Here's how the part is built. I have some questions about the finished solid (model axes, mm). Face numbers are marked on the shaded views. Give positions to 0.01 mm unless a question says otherwise; leave off trailing zeros. Write each loop counter-clockwise with the first axis right and the second up, starting at its lowest first coordinate (ties: lowest second). Pieces come first, ordered by that corner, then holes. Notation, with made-up numbers: (43.5, -4) - (68.5, -4) arc R30 cw to (68.5, 33) - close; hole circle Ø5 at (50.25, 49). An arc over 180 degrees is marked (long way). One line per item, written item: value. Start each with the question number.
1) Imagine slicing it at A-A on y = -10.5. Write out the boundary of the cut face in (x, z), plus the area to 3 significant figures.
2) Imagine slicing it at B-B on x = 27.5. Write out the boundary of the cut face in (y, z), plus the area to 3 significant figures.
3) Please list where these lines run through material, in increasing order: L1, parallel to Y at x = -64.5, z = 0.5; L2, parallel to Y at x = 27.5, z = 1; L3, parallel to Y at x = -64.5, z = 1.5. Write a range as [from, to].
4) Imagine slicing it at C-C on z = -1.2. Write out the boundary of the cut face in (x, y), plus the area to 3 significant figures.
5) We'd pull the mould along X, two halves only. Please class the marked faces 1 and 2: +X half, -X half, draft (parallel to the pull), parting line (faces both ways), or undercut.
6) I'm going to push a flat-ended pin straight in: P1, Ø8, axis at x = 54.5, y = -4.5, coming from the -Z side. Where does the tip first touch, or does it pass through?
7) Imagine slicing it at D-D on x = 6. Write out the boundary of the cut face in (y, z), plus the area to 3 significant figures.
from build123d import *

# Parameters (mm, degrees)
F0_W     = 166
F0_H     = 70
F1_DEPTH = 2
F2_W     = 77
F2_H     = 33.5
F2_R     = 2.1
F2_R_2   = 8.25
F3_DEPTH = 2
F4_R     = 1.5
F5_DEPTH = 3
F6_SIZE  = 1
F7_SIZE  = 1


with BuildPart() as f1:
    # F0 (on Top) → F1 (new body)
    with BuildSketch(Plane.XY):
        Rectangle(F0_W, F0_H)
    extrude(amount=F1_DEPTH)

    # F2 (on face) → F3 (cut, through all)
    with BuildSketch(Plane.XY.offset(2)):
        with Locations((-29.25, 1.5)):
            Rectangle(F2_W, F2_H)
        with Locations((-64.5, 21.5)):
            Circle(F2_R)
        with Locations((6, 21.5)):
            Circle(F2_R)
        with Locations((6, -18.5)):
            Circle(F2_R)
        with Locations((-64.5, -18.5)):
            Circle(F2_R)
        with Locations((27.5, 1.5)):
            Circle(F2_R_2)
        with Locations((57.5, 1.5)):
            Circle(F2_R_2)
    extrude(amount=-F3_DEPTH, mode=Mode.SUBTRACT)

    # F4 (on face) → F5 (join)
    with BuildSketch(Plane(origin=(0, 0, 0), x_dir=(1, 0, 0), z_dir=(0, 0, -1))):
        with Locations((-79.5, 30)):
            Circle(F4_R)
        with Locations((-79.5, -30)):
            Circle(F4_R)
        with Locations((-79.5, 0)):
            Circle(F4_R)
        with Locations((79.5, -30)):
            Circle(F4_R)
        with Locations((79.5, 30)):
            Circle(F4_R)
        with Locations((79.5, 0)):
            Circle(F4_R)
    extrude(amount=F5_DEPTH)

    # F6
    f6_edges = [f1.edges().sort_by_distance(p)[0] for p in [
        (-81, -30, -3),
        (-81, 0, -3),
        (-81, 30, -3),
        (78, 30, -3),
        (78, 0, -3),
        (78, -30, -3),
    ]]
    chamfer(f6_edges, length=F6_SIZE)

    # F7
    f7_edges = [f1.edges().sort_by_distance(p)[0] for p in [
        (83, 0, 2),
        (0, -35, 2),
        (-83, 0, 2),
        (0, 35, 2),
    ]]
    chamfer(f7_edges, length=F7_SIZE)


solid = f1.part
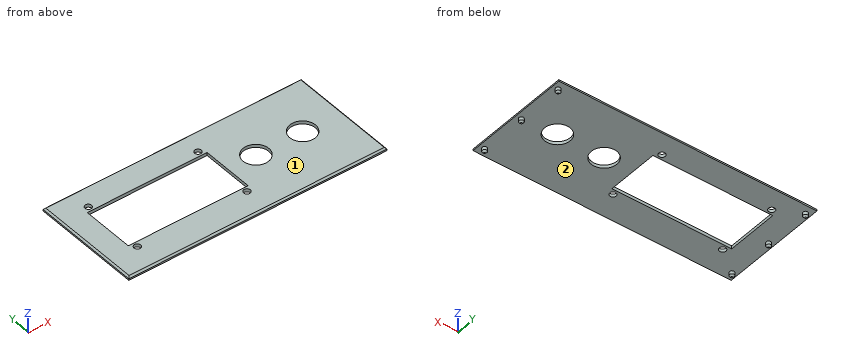
Numbers:
1. outline: (-83, 0) - (-67.75, 0) - (-67.75, 2) - (-82, 2) - (-83, 1) - close; (9.25, 0) - (83, 0) - (83, 1) - (82, 2) - (9.25, 2) - close
1. area: 177 mm^2
2. outline: (-35, 0) - (-6.75, 0) - (-6.75, 2) - (-34, 2) - (-35, 1) - close; (9.75, 0) - (35, 0) - (35, 1) - (34, 2) - (9.75, 2) - close
2. area: 106 mm^2
3. L1: [-35, -20.6], [-16.4, -15.25], [18.25, 19.4], [23.6, 35]
3. L2: [-35, -6.75], [9.75, 35]
3. L3: [-34.5, -20.6], [-16.4, -15.25], [18.25, 19.4], [23.6, 34.5]
4. outline: circle Ø3 at (-79.5, -30); circle Ø3 at (-79.5, 0); circle Ø3 at (-79.5, 30); circle Ø3 at (79.5, -30); circle Ø3 at (79.5, 0); circle Ø3 at (79.5, 30)
4. area: 42.4 mm^2
5. face 1: draft
5. face 2: undercut
6. P1: z = 0
7. outline: (-35, 0) - (-20.6, 0) - (-20.6, 2) - (-34, 2) - (-35, 1) - close; (-16.4, 0) - (-15.25, 0) - (-15.25, 2) - (-16.4, 2) - close; (18.25, 0) - (19.4, 0) - (19.4, 2) - (18.25, 2) - close; (23.6, 0) - (35, 0) - (35, 1) - (34, 2) - (23.6, 2) - close
7. area: 55.2 mm^2
